Check sheet for the modelled part. Datum: model origin and axes. Units: mm. Round coordinates to 2 decimals unless told otherwise and drop trailing zeros. Write each loop counter-clockwise with the first axis right and the second up, starting at its lowest first coordinate (ties: lowest second). Pieces come first, ordered by that corner, then holes.
Item 1: Material ranges on line 1 (X direction, y = 1.55, z = 0); line 2 (X direction, y = 0.1, z = -1.25); line 3 (Z direction, x = 24, y = 1.45), recorded low to high.
Item 2: Cross-section at B-B on y = 1.2. Count the separate pieces of the cut face and the enclosed holes in it, plus the area to 3 significant figures.
Item 3: Go/stop test with flat-tipped pins: pin 1 Ø2.5 at (x, z) = (-28.05, 0) entering from -Y; pin 2 Ø0.6 at (x, y) = (26.5, 1) entering from -Z; pin 3 Ø1 at (y, z) = (1.5, -2.5) entering from -X; pin 4 Ø0.6 at (x, y) = (-26.5, 0.5) entering from +Z. Record where each tip stops, or that it passes through.
Item 4: Cross-section at A-A on z = 0. Enter the section's corners in (x, y).
from build123d import *

# Parameters (mm, degrees)
SKETCH1_R           = 1.5
BOSS_EXTRUDE1_DEPTH = 2
FILLET1_R           = 3
FILLET2_R           = 1


with BuildPart() as part:
    # Sketch1 → Boss-Extrude1 (new body)
    with BuildSketch(Plane(origin=(0, 0, 0), x_dir=(1, 0, 0), z_dir=(0, 1, 0))):
        Polygon((-23.75, 5), (23.65, 5), (23.65, 4), (30.95, 4), (30.95, -4), (23.65, -4), (23.65, -5), (-23.75, -5), (-23.75, -4), (-31.05, -4), (-31.05, 4), (-23.75, 4), align=None)
        with Locations(Location((-28.05, 0, 0), (0, 0, 270))):
            Circle(SKETCH1_R, mode=Mode.SUBTRACT)
        with Locations(Location((27.95, 0, 0), (0, 0, 270))):
            Circle(SKETCH1_R, mode=Mode.SUBTRACT)
    extrude(amount=BOSS_EXTRUDE1_DEPTH)

    # Fillet1
    fillet1_edges = [part.edges().sort_by_distance(p)[0] for p in [
        (-31.05, 1, -4),
        (30.95, 1, -4),
    ]]
    fillet(fillet1_edges, radius=FILLET1_R)

    # Fillet2
    fillet2_edges = [part.edges().sort_by_distance(p)[0] for p in [
        (-23.75, 1, 5),
        (23.65, 1, 5),
        (23.65, 1, -5),
        (-23.75, 1, -5),
        (-31.05, 1, 4),
        (30.95, 1, 4),
    ]]
    fillet(fillet2_edges, radius=FILLET2_R - 0.0001)  # a hair under: the kernel refuses the full size


solid = part.part
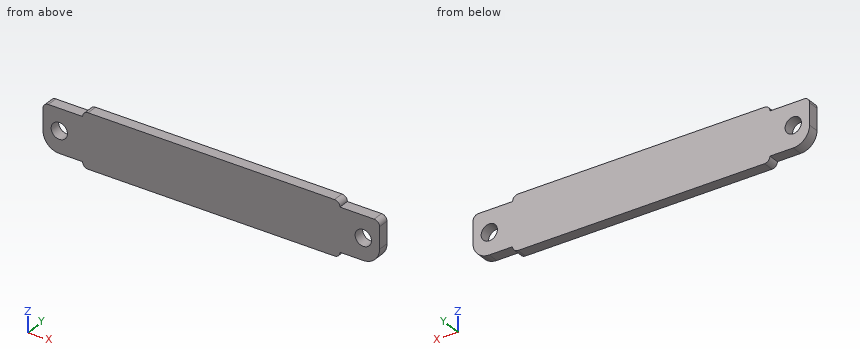
Response values:
1. line 1: x = -31.05 to -29.55, -26.55 to 26.45, 29.45 to 30.95
1. line 2: x = -31.04 to -28.88, -27.22 to 27.12, 28.78 to 30.94
1. line 3: z = -4 to 4
2. separate pieces: 1
2. enclosed holes: 2
2. area: 572 mm2
3. pin 1: passes through
3. pin 2: stops at z = -4
3. pin 3: stops at x = -30.88
3. pin 4: stops at z = 4
4. outline: (-31.05, 0) - (-29.55, 0) - (-29.55, 2) - (-31.05, 2) - close; (-26.55, 0) - (26.45, 0) - (26.45, 2) - (-26.55, 2) - close; (29.45, 0) - (30.95, 0) - (30.95, 2) - (29.45, 2) - close
